Can you work these out from the model? Positions are in its coordinate system, mm. A direction names the side the tool comes from. Round coordinates to 2 decimals unless told otherwise and drop trailing zeros. Loops run counter-clockwise (first coordinate to the right, second up) from the corner with the lowest first, then second, coordinate; pieces in that order, holes last.
(1) Will these pins go through, and if not, where does the flat tip stop? pin 1 Ø1 at (x, y) = (-51, -43) entering from +Z; pin 2 Ø3.5 at (y, z) = (25.5, 126.5) entering from -X; pin 3 Ø1.5 at (y, z) = (14.5, 125) entering from +X.
(2) Which directions (+Z, -Z, +X, -X, +Y, -Y) give clear straight access to the entire face, cutting with the end or side of a thin tool? Please do faces 1 (the face through (83.237, -1, 61)), 2 (the face through (86.237, -1, 63)).
(3) I want a section at B-B on y = -65.5. Write out the boundary of the cut face in (x, z).
(4) I want a section at A-A on z = 102.5. Write out the boundary of the cut face in (x, y).
(5) I want a section at C-C on x = -53. Write out the boundary of the cut face in (y, z), plus the area to 3 significant figures.
(6) If I drill on line 1 along X through (y, z) = (-50, 82); line 2 along Z through (x, y) = (-69, 4); line 3 along X through (y, z) = (-40.55, 125.95), over which ranges is the centre line in solid material (lowest first)?
(7) Thinking about a two-plate mould opening in X: for faces 3 (the face through (-86.237, -1, 61)), 4 (the face through (70, -1, 127.223)), 5 (the face through (-83.237, -1, 63)), 6 (the face through (-69, 1, 124.223)), which applies, released by +X, released by -X, zero draft, split by the parting line, or undercut?
from build123d import *

# Parameters (mm, degrees)
SKETCH1_W                    = 165
SKETCH1_H                    = 200
BASE_FLANGE1_DEPTH           = 3
SKETCH6_W                    = 130
SKETCH6_H                    = 200
TAB1_DEPTH                   = 3
SKETCHED_START               = -100
SKETCHED_BEND1_DEPTH         = 200
SKETCHED_BEND1_2_DEPTH       = 200
SKETCH10_W                   = 130
SKETCH10_H                   = 200
TAB2_DEPTH                   = 3
SKETCHED_BEND2_DEPTH         = 200
SKETCHED_BEND2_2_DEPTH       = 200
EDGE_FLANGE1_STRIP_W         = 13.4732
EDGE_FLANGE1_STRIP_H         = 3
EDGE_FLANGE1_STRIP_CUT_DEPTH = 200
EDGE_FLANGE1_DEPTH           = 200
EDGE_FLANGE2_STRIP_W         = 13.4732
EDGE_FLANGE2_STRIP_H         = 3
EDGE_FLANGE2_STRIP_CUT_DEPTH = 200
EDGE_FLANGE2_DEPTH           = 200
SKETCH20_R                   = 1.75
CUT_EXTRUDE1_DEPTH           = 10


# Read off the part's stored shape, not the designer's step: Sketched Bend1, Sketched Bend2
# Sheet-metal steps are written as plain solids
with BuildPart() as part:
    # Sketch1 → Base-Flange1 (new body)
    with BuildSketch(Plane.XY):
        Rectangle(SKETCH1_W, SKETCH1_H)
    extrude(amount=-BASE_FLANGE1_DEPTH)

    # Sketch6 → Tab1 (add)
    with BuildSketch(Plane(origin=(0, 0, -3), x_dir=(-1, 0, 0), z_dir=(0, 0, -1))):
        with Locations((-147.5, 0)):
            Rectangle(SKETCH6_W, SKETCH6_H)
    extrude(amount=-TAB1_DEPTH)

    # Sketched Bend1 outline → Sketched Bend1 (cut)
    with BuildSketch(Plane(origin=(0, 0, 0), x_dir=(1, 0, 0), z_dir=(0, 1, 0)).offset(SKETCHED_START)):
        with BuildLine():
            ThreePointArc((82.5, 3), (84.867467001, 2.154295979), (86.163277222, 0))
            Line((86.163277222, 0), (212.5, 0))
            Line((212.5, 0), (212.5, 3))
            Line((212.5, 3), (82.5, 3))
        make_face()
    extrude(amount=SKETCHED_BEND1_DEPTH, mode=Mode.SUBTRACT)

    # Sketched Bend1 2 outline → Sketched Bend1 2 (add)
    with BuildSketch(Plane(origin=(0, 0, 0), x_dir=(1, 0, 0), z_dir=(0, 1, 0)).offset(SKETCHED_START)):
        with BuildLine():
            Line((86.2366, -127.223356935), (86.2366, -0.7366))
            ThreePointArc((86.2366, -0.7366), (86.218224121, -0.36647982), (86.163277222, 0))
            Line((86.163277222, 0), (82.5, 0))
            ThreePointArc((82.5, 0), (83.020854855, -0.215745145), (83.2366, -0.7366))
            Line((83.2366, -0.7366), (83.2366, -127.223356935))
            Line((83.2366, -127.223356935), (86.2366, -127.223356935))
        make_face()
    extrude(amount=SKETCHED_BEND1_2_DEPTH)

    # Sketch10 → Tab2 (add)
    with BuildSketch(Plane.XY):
        with Locations((-147.5, 0)):
            Rectangle(SKETCH10_W, SKETCH10_H)
    extrude(amount=-TAB2_DEPTH)

    # Sketched Bend2 outline → Sketched Bend2 (cut)
    with BuildSketch(Plane(origin=(0, 0, 0), x_dir=(1, 0, 0), z_dir=(0, 1, 0)).offset(SKETCHED_START)):
        with BuildLine():
            Line((-212.5, 0), (-86.163277222, 0))
            ThreePointArc((-86.163277222, 0), (-84.867467001, 2.154295979), (-82.5, 3))
            Line((-82.5, 3), (-212.5, 3))
            Line((-212.5, 3), (-212.5, 0))
        make_face()
    extrude(amount=SKETCHED_BEND2_DEPTH, mode=Mode.SUBTRACT)

    # Sketched Bend2 2 outline → Sketched Bend2 2 (add)
    with BuildSketch(Plane(origin=(0, 0, 0), x_dir=(1, 0, 0), z_dir=(0, 1, 0)).offset(SKETCHED_START)):
        with BuildLine():
            Line((-86.2366, -0.7366), (-86.2366, -127.223356935))
            Line((-86.2366, -127.223356935), (-83.2366, -127.223356935))
            Line((-83.2366, -127.223356935), (-83.2366, -0.7366))
            ThreePointArc((-83.2366, -0.7366), (-83.020854855, -0.215745145), (-82.5, 0))
            Line((-82.5, 0), (-86.163277222, 0))
            ThreePointArc((-86.163277222, 0), (-86.218224121, -0.36647982), (-86.2366, -0.7366))
        make_face()
    extrude(amount=SKETCHED_BEND2_2_DEPTH)

    # Edge-Flange1 strip (across the edge) → Edge-Flange1 strip cut (cut)
    with BuildSketch(Plane(origin=(-83.2366, 100, 127.223356935), x_dir=(0, 0, -1), z_dir=(0, -1, 0))):
        with Locations((-3, -1.5)):
            Rectangle(EDGE_FLANGE1_STRIP_W, EDGE_FLANGE1_STRIP_H)
    extrude(amount=EDGE_FLANGE1_STRIP_CUT_DEPTH, mode=Mode.SUBTRACT)

    # Edge-Flange1 section (across the edge) → Edge-Flange1 (add)
    with BuildSketch(Plane(origin=(-83.2366, 100, 127.223356935), x_dir=(0, 0, -1), z_dir=(0, -1, 0))):
        with BuildLine():
            Line((0, 0.7366), (0, 27))
            Line((0, 27), (3, 27))
            Line((3, 27), (3, 0.7366))
            ThreePointArc((3, 0.7366), (3.215745145, 0.215745145), (3.7366, 0))
            Line((3.7366, 0), (3.7366, -3))
            ThreePointArc((3.7366, -3), (1.094424801, -1.905575199), (0, 0.7366))
        make_face()
    extrude(amount=EDGE_FLANGE1_DEPTH)

    # Edge-Flange2 strip (across the edge) → Edge-Flange2 strip cut (cut)
    with BuildSketch(Plane(origin=(83.2366, -100, 127.223356935), x_dir=(0, 0, -1), z_dir=(0, 1, 0))):
        with Locations((-3, -1.5)):
            Rectangle(EDGE_FLANGE2_STRIP_W, EDGE_FLANGE2_STRIP_H)
    extrude(amount=EDGE_FLANGE2_STRIP_CUT_DEPTH, mode=Mode.SUBTRACT)

    # Edge-Flange2 section (across the edge) → Edge-Flange2 (add)
    with BuildSketch(Plane(origin=(83.2366, -100, 127.223356935), x_dir=(0, 0, -1), z_dir=(0, 1, 0))):
        with BuildLine():
            Line((0, 0.7366), (0, 27))
            Line((0, 27), (3, 27))
            Line((3, 27), (3, 0.7366))
            ThreePointArc((3, 0.7366), (3.215745145, 0.215745145), (3.7366, 0))
            Line((3.7366, 0), (3.7366, -3))
            ThreePointArc((3.7366, -3), (1.094424801, -1.905575199), (0, 0.7366))
        make_face()
    extrude(amount=EDGE_FLANGE2_DEPTH)

    # Sketch20 → Cut-Extrude1 (cut)
    with BuildSketch(Plane(origin=(0, 0, 124.223356935), x_dir=(-1, 0, 0), z_dir=(0, 0, -1))):
        with Locations(Location((-60.9866, -40.55, 0), (0, 0, 90))):
            Circle(SKETCH20_R)
        with Locations(Location((60.9866, -40.55, 0), (0, 0, 90))):
            Circle(SKETCH20_R)
    extrude(amount=-CUT_EXTRUDE1_DEPTH, mode=Mode.SUBTRACT)


solid = part.part
Filled sheet:
1. pin 1: stops at z = 0
1. pin 2: stops at x = -86.02
1. pin 3: stops at x = 86.16
2. face 1: +Y, -Y
2. face 2: +Z, -Z, +X, +Y, -Y
3. outline: (-86.24, 0.74) arc R3.74 ccw to (-82.5, -3) - (82.5, -3) arc R3.74 ccw to (86.24, 0.74) - (86.24, 123.49) arc R3.74 ccw to (82.5, 127.22) - (56.24, 127.22) - (56.24, 124.22) - (82.5, 124.22) arc R0.74 cw to (83.24, 123.49) - (83.24, 0.74) arc R0.74 cw to (82.5, 0) - (-82.5, 0) arc R0.74 cw to (-83.24, 0.74) - (-83.24, 123.49) arc R0.74 cw to (-82.5, 124.22) - (-56.24, 124.22) - (-56.24, 127.22) - (-82.5, 127.22) arc R3.74 ccw to (-86.24, 123.49) - close
4. outline: (-86.24, -100) - (-83.24, -100) - (-83.24, 100) - (-86.24, 100) - close; (83.24, -100) - (86.24, -100) - (86.24, 100) - (83.24, 100) - close
5. outline: (-100, -3) - (100, -3) - (100, 0) - (-100, 0) - close
5. area: 600 mm2
6. line 1: x = -86.24 to -83.24, 83.24 to 86.24
6. line 2: z = -3 to 0, 124.22 to 127.22
6. line 3: x = -85.31 to -62.74, -59.24 to -56.24, 56.24 to 59.24, 62.74 to 85.31
7. face 3: released by -X
7. face 4: zero draft
7. face 5: undercut
7. face 6: undercut
